Build history of the part. All positions in model axes, mm. A direction names the side the tool comes from. Give positions to 0.01 mm unless a question says otherwise; leave off trailing zeros. Order: outer loops, then holes, each group sorted by start corner. A loop starts at its lowest first (then second) coordinate and runs counter-clockwise, first axis right, second up. Notation, with made-up numbers: (-37, 63.25) - (16, 63.25) arc R20 cw to (16, 70.25) - close; hole circle Ø5 at (-30, 35). An arc over 180 degrees is marked (long way). Use a Markdown table: item, result.
from build123d import *

# Parameters (mm, degrees)
EXTRUDE1_DEPTH         = 95.25
SKETCH2_R              = 6.731
CUT_CHAMFER_DEPTH      = 508
CUT_CHAMFER_DEPTH_BACK = 58.15
SKETCH3_R              = 6.746875
CUT_HOLES_DEPTH        = 229.6


with BuildPart() as part:
    # Sketch1 → Extrude1 (new body, symmetric)
    with BuildSketch(Plane.XY):
        with BuildLine():
            Line((228.6, 0), (15.875, 0))
            ThreePointArc((15.875, 0), (4.649679849, -4.649679849), (0, -15.875))
            Line((0, -15.875), (0, -57.15))
            Line((0, -57.15), (6.35, -57.15))
            Line((6.35, -57.15), (6.35, -15.875))
            ThreePointArc((6.35, -15.875), (9.139807909, -9.139807909), (15.875, -6.35))
            Line((15.875, -6.35), (228.6, -6.35))
            Line((228.6, -6.35), (228.6, 0))
        make_face()
    extrude(amount=EXTRUDE1_DEPTH, both=True)

    # Sketch2 → Cut-Chamfer (cut, two sides)
    with BuildSketch(Plane(origin=(0, 0, 0), x_dir=(1, 0, 0), z_dir=(0, 1, 0))) as cut_chamfer_sk:
        with Locations((209.55, 0)):
            Circle(SKETCH2_R)
        with Locations((139.7, 0)):
            Circle(SKETCH2_R)
        Polygon((25.4, 95.25), (228.6, 25.4), (228.6, 95.25), align=None)
        Polygon((25.4, -95.25), (228.6, -25.4), (228.6, -95.25), align=None)
    extrude(amount=CUT_CHAMFER_DEPTH, mode=Mode.SUBTRACT)
    extrude(cut_chamfer_sk.sketch, amount=-CUT_CHAMFER_DEPTH_BACK, mode=Mode.SUBTRACT)

    # Sketch3 → Cut-Holes (cut, through all)
    with BuildSketch(Plane(origin=(0, 0, 0), x_dir=(0, 0, -1), z_dir=(1, 0, 0))):
        with Locations((-76.2, -36.5125)):
            Circle(SKETCH3_R)
        with Locations((76.2, -36.5125)):
            Circle(SKETCH3_R)
    extrude(amount=CUT_HOLES_DEPTH, mode=Mode.SUBTRACT)


solid = part.part
1) Tool access for faces 1 (the flat face through (6.35, -37, 1)), 2 (the flat face through (125.578, -3.131, 60.814)): list every direction of +Z, -Z, +X, -X, +Y, -Y with a clear straight run to the whole face (end or side of a thin tool).
Computed:
| item | result |
|---|---|
| face 1 | +Z, -Z, +X, -Y |
| face 2 | +Z, +X, +Y, -Y |
2) Slice it at B-B (y = -32.5). Write the cut outline in (x, z).
Computed:
| item | result |
|---|---|
| outline | (0, -95.25) - (6.35, -95.25) - (6.35, -81.62) - (0, -81.62) - close; (0, -70.78) - (6.35, -70.78) - (6.35, 70.78) - (0, 70.78) - close; (0, 81.62) - (6.35, 81.62) - (6.35, 95.25) - (0, 95.25) - close |
3) Slice it at D-D (z = -76.2). Write the cut outline in (x, y) (3 decimals).
Computed:
| item | result |
|---|---|
| outline | (0, -57.15) - (6.35, -57.15) - (6.35, -43.259) - (0, -43.259) - close; (0, -29.766) - (6.35, -29.766) - (6.35, -15.875) arc R9.525 cw to (15.875, -6.35) - (80.818, -6.35) - (80.818, 0) - (15.875, 0) arc R15.875 ccw to (0, -15.875) - close |
4) Slice it at A-A (z = -15.5). Write the cut outline in (x, y) (3 decimals).
Computed:
| item | result |
|---|---|
| outline | (0, -57.15) - (6.35, -57.15) - (6.35, -15.875) arc R9.525 cw to (15.875, -6.35) - (228.6, -6.35) - (228.6, 0) - (15.875, 0) arc R15.875 ccw to (0, -15.875) - close |
5) Slice it at C-C (x = 139.7). Write the cut outline in (y, z).
Computed:
| item | result |
|---|---|
| outline | (-6.35, -55.96) - (0, -55.96) - (0, -6.73) - (-6.35, -6.73) - close; (-6.35, 6.73) - (0, 6.73) - (0, 55.96) - (-6.35, 55.96) - close |
6) Pin check, flat tips, straight feed: P1, Ø1.5, axis at x = 86.5, z = 0.5, coming from the -Y side; P2, Ø20.5, axis at y = -35.5, z = 16, coming from the +X side. Stop position of each tip, or through.
Computed:
| item | result |
|---|---|
| P1 | stops at y = -6.35 |
| P2 | stops at x = 6.35 |
7) Wall check: line 1 (Y direction, x = 130, z = 4.5); line 2 (X direction, y = -23.5, z = -2); line 3 (X direction, y = -4.5, z = 0). Give the ranges that are in metal, low to high. Write a range as from..to.
Computed:
| item | result |
|---|---|
| line 1 | y = -6.35..0 |
| line 2 | x = 0..6.35 |
| line 3 | x = 4.8..132.97, 146.43..202.82, 216.28..228.6 |
8) Two-plate mould, pull along Z, no slides. Class faces 3 (the flat face through (6, -24, -95.25)), 4 (the cylindrical face through (215.97, -3.13, -2.02)), 5 (the flat face through (97, -6.35, 1)): +Z half, -Z half, draft (parallel to the pull), parting line (faces both ways), or undercut.
Computed:
| item | result |
|---|---|
| face 3 | -Z half |
| face 4 | undercut |
| face 5 | draft |
